The figure shows three views and two pictorial views of one solid part (mm, origin at its lowest corner). Answer the questions. A direction names the side the tool comes from. Coordinates: 2 decimals unless noted, no trailing zeros. Loops run counter-clockwise (first coordinate to the right, second up) from the corner with the lowest first, then second, coordinate; pieces in that order, holes last. Notation, with made-up numbers: M -5.75,-1.5 L 23.25,-1.5 A27 cw 23.25,28.5 Z; hole C 59.5,50.25 d11. An arc over 180 degrees is marked long. Return JSON: item names as keys, results as strings. Group by question number.
1. Section C-C (y = 8) is taken. Write down the section's boundary in (x, z).
2. Which of the six approach directions +Z, -Z, +X, -X, +Y, -Y give full straight-line access (tool end or side, diameter ignored) to the marked faces 1, 2 and 3?
3. Straight lines are drawn through the part: L1, parallel to Y at x = 5, z = 11.3; L2, parallel to Z at x = 30, y = 3.5; L3, parallel to X at y = 1.3, z = 6 (1 decimal). For each, find the intervals that lie inside material, in ascending order. Write a range as from..to.
4. Section B-B (x = 20.5) is taken. Write down the section's boundary in (y, z), then the cut area to 3 significant figures.
5. Given P1, Ø2, axis at y = 9, z = 8.5, coming from the -X side; P2, Ø4, axis at x = 13, z = 3.5, coming from the +Y side; P3, Ø3, axis at x = 19, z = 5, coming from the +Y side, each flat-ended and moving along its own axis, determine where each tip first touches the part or whether it passes through.
6. The mould has two halves that part along X. Classify the marked faces 4, 5 and 6: pulls with the +X half, pulls with the -X half, needs draft (parallel to the pull), parting line crosses it, or undercut.
7. Section A-A (z = 6) is taken. Count the separate pieces of the cut face and the enclosed holes in it, then the cut area to 3 significant figures.
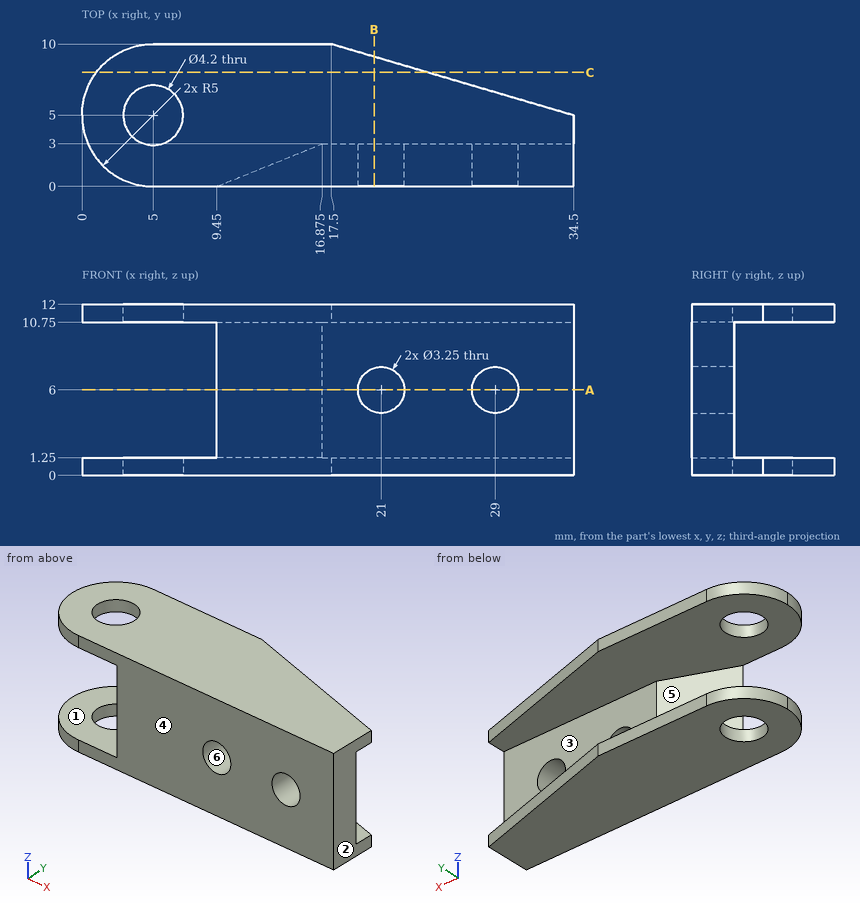
Worked out:
{
 "1": {"outline": "M 1,0 L 24.3,0 L 24.3,1.25 L 1,1.25 Z; M 1,10.75 L 24.3,10.75 L 24.3,12 L 1,12 Z"},
 "2": {"face 1": "-X, +Y", "face 2": "+Z, -Z, +X, +Y, -Y", "face 3": "+X, -X, +Y"},
 "3": {"L1": "0..2.9, 7.1..10", "L2": "0..1.25, 10.75..12", "L3": "12.7..19.4, 22.6..27.4, 30.6..34.5"},
 "4": {"outline": "M 0,0 L 9.12,0 L 9.12,1.25 L 3,1.25 L 3,4.45 L 0,4.45 Z; M 0,7.55 L 3,7.55 L 3,10.75 L 9.12,10.75 L 9.12,12 L 0,12 Z", "area": "42.0 mm^2"},
 "5": {"P1": "through", "P2": "y = 2.24", "P3": "y = 3"},
 "6": {"face 4": "needs draft", "face 5": "pulls with the -X half", "face 6": "undercut"},
 "7": {"separate pieces": "3", "enclosed holes": "0", "area": "44.5 mm^2"}
}
